Could you check a few things on this drawing? It's one solid part, dimensions in mm from its lowest x, y, z. Give positions to 0.01 mm unless a question says otherwise; leave off trailing zeros. Loops run counter-clockwise (first coordinate to the right, second up) from the corner with the lowest first, then second, coordinate; pieces in that order, holes last. Notation, with made-up numbers: M 89,27 L 120,27 A30 ccw 120,62 Z; hole C -34.75,15 d10. An arc over 180 degrees is marked long. Answer in a Markdown table with one row per item. Add a question column.
1. I need wall thicknesses on line 1 along X through (y, z) = (0.5, 5); line 2 along Y through (x, z) = (12, 7); line 3 along Z through (x, y) = (10.75, 1.15). Which ranges of each line are inside material? Lowest first, please. Write a range as from..to.
2. If we section it at C-C on z = 1.25: List the corners of the cut face in (x, y) for me.
3. If we section it at A-A on z = 5: List the corners of the cut face in (x, y) for me.
4. Thinking about a two-plate mould opening in X: for the marked faces 1, 2 and 3, which applies, released by +X, released by -X, zero draft, split by the parting line, or undercut?
5. If we section it at D-D on y = 1: List the corners of the cut face in (x, z) for me.
6. I'm going to push flat-ended pins straight in: pin 1 Ø3 at (x, z) = (9, 4.5) entering from +Y; pin 2 Ø3.5 at (x, z) = (9.57, 5) entering from -Y. Where does each tip first touch, or does it pass through?
7. If we section it at B-B on x = 10.75: List the corners of the cut face in (y, z) for me.
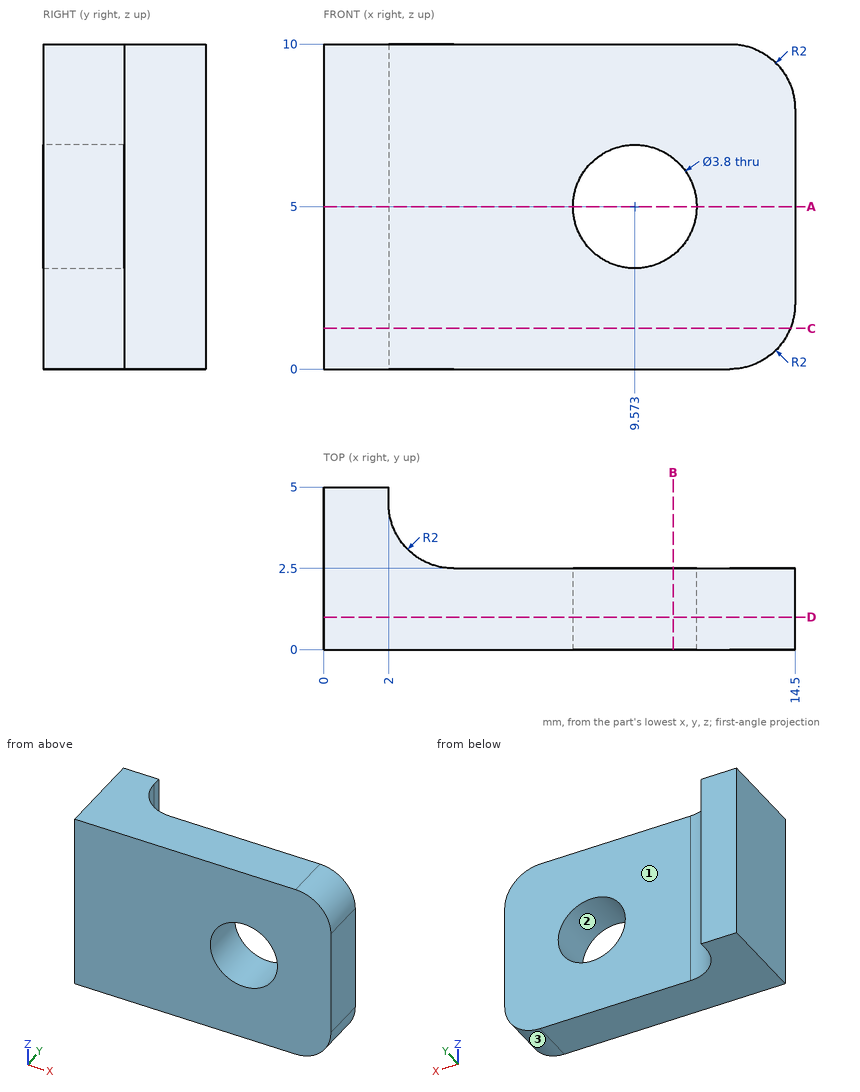
Results:
| question | item | result |
|---|---|---|
| 1 | line 1 | 0..7.67, 11.47..14.5 |
| 1 | line 2 | 0..2.5 |
| 1 | line 3 | 0..3.51, 6.49..10 |
| 2 | outline | M 0,0 L 14.35,0 L 14.35,2.5 L 4,2.5 A2 cw 2,4.5 L 2,5 L 0,5 Z |
| 3 | outline | M 0,0 L 7.67,0 L 7.67,2.5 L 4,2.5 A2 cw 2,4.5 L 2,5 L 0,5 Z; M 11.47,0 L 14.5,0 L 14.5,2.5 L 11.47,2.5 Z |
| 4 | face 1 | zero draft |
| 4 | face 2 | undercut |
| 4 | face 3 | released by +X |
| 5 | outline | M 0,0 L 12.5,0 A2 ccw 14.5,2 L 14.5,8 A2 ccw 12.5,10 L 0,10 Z; hole C 9.57,5 d3.8 |
| 6 | pin 1 | y = 2.5 |
| 6 | pin 2 | through |
| 7 | outline | M 0,0 L 2.5,0 L 2.5,3.51 L 0,3.51 Z; M 0,6.49 L 2.5,6.49 L 2.5,10 L 0,10 Z |
